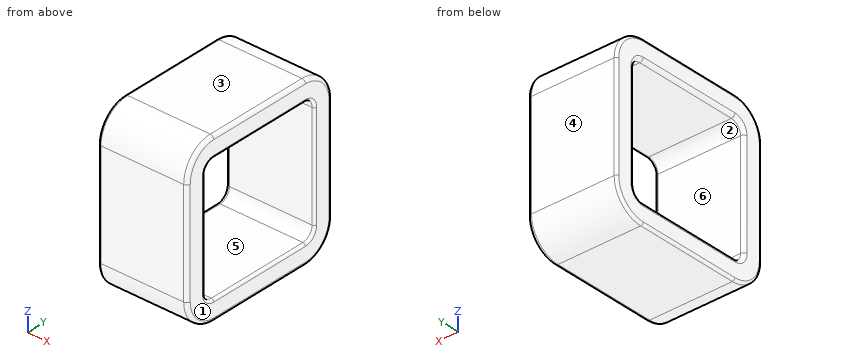
```python
from build123d import *

# Parameters (mm, degrees)
BOSS_EXTRUDE1_DEPTH      = 12
BOSS_EXTRUDE1_DEPTH_BACK = 5.8
FILLET2_R                = 0.7
FILLET3_R                = 0.5


with BuildPart() as part:
    # Sketch1 → Boss-Extrude1 (new, two sides: drawn at the far end of the back side and taken through both)
    with BuildSketch(Plane(origin=(72.6, 0, 0), x_dir=(0, 0, -1), z_dir=(1, 0, 0)).offset(-BOSS_EXTRUDE1_DEPTH_BACK)):
        with BuildLine():
            Line((-31.6, 17.5), (-31.6, -3.5))
            ThreePointArc((-31.6, -3.5), (-29.813351365, -7.813351365), (-25.5, -9.6))
            Line((-25.5, -9.6), (-4.5, -9.6))
            ThreePointArc((-4.5, -9.6), (-0.186648635, -7.813351365), (1.6, -3.5))
            Line((1.6, -3.5), (1.6, 17.5))
            ThreePointArc((1.6, 17.5), (-0.186648635, 21.813351365), (-4.5, 23.6))
            Line((-4.5, 23.6), (-25.5, 23.6))
            ThreePointArc((-25.5, 23.6), (-29.813351365, 21.813351365), (-31.6, 17.5))
        make_face()
        with BuildLine():
            Line((-27.6, 17.5), (-27.6, -3.5))
            ThreePointArc((-27.6, -3.5), (-26.98492424, -4.98492424), (-25.5, -5.6))
            Line((-25.5, -5.6), (-4.5, -5.6))
            ThreePointArc((-4.5, -5.6), (-3.01507576, -4.98492424), (-2.4, -3.5))
            Line((-2.4, -3.5), (-2.4, 17.5))
            ThreePointArc((-2.4, 17.5), (-3.01507576, 18.98492424), (-4.5, 19.6))
            Line((-4.5, 19.6), (-25.5, 19.6))
            ThreePointArc((-25.5, 19.6), (-26.98492424, 18.98492424), (-27.6, 17.5))
        make_face(mode=Mode.SUBTRACT)
    extrude(amount=BOSS_EXTRUDE1_DEPTH + BOSS_EXTRUDE1_DEPTH_BACK)

    # Fillet2
    fillet2_edges = [part.edges().sort_by_distance(p)[0] for p in [
        (66.8, 18.98492424, 26.98492424),
        (66.8, 7, 27.6),
        (66.8, -4.98492424, 26.98492424),
        (66.8, -5.6, 15),
        (84.6, 23.6, 15),
        (66.8, -4.98492424, 3.01507576),
        (66.8, 18.98492424, 3.01507576),
        (84.6, 21.813351365, 29.813351365),
        (66.8, 7, 2.4),
        (66.8, 19.6, 15),
        (84.6, 7, 31.6),
        (84.6, -7.813351365, 29.813351365),
        (84.6, -9.6, 15),
        (84.6, -7.813351365, 0.186648635),
        (84.6, 7, -1.6),
        (84.6, 21.813351365, 0.186648635),
    ]]
    fillet(fillet2_edges, radius=FILLET2_R)

    # Fillet3
    fillet3_edges = [part.edges().sort_by_distance(p)[0] for p in [
        (84.6, 19.6, 15),
        (84.6, 18.98492424, 3.01507576),
        (84.6, 7, 2.4),
        (84.6, -4.98492424, 3.01507576),
        (84.6, -5.6, 15),
        (84.6, -4.98492424, 26.98492424),
        (84.6, 7, 27.6),
        (66.8, 23.6, 15),
        (66.8, 7, -1.6),
        (66.8, 21.813351365, 0.186648635),
        (66.8, -7.813351365, 0.186648635),
        (66.8, -9.6, 15),
        (66.8, -7.813351365, 29.813351365),
        (66.8, 7, 31.6),
        (66.8, 21.813351365, 29.813351365),
        (84.6, 18.98492424, 26.98492424),
    ]]
    fillet(fillet3_edges, radius=FILLET3_R)


solid = part.part
```
The listing builds one solid part. Answer for the finished solid, in the listing's coordinates (mm). Face numbers are marked on the shaded views. A direction names the side the tool comes from. Give positions to 0.01 mm unless a question says otherwise; leave off trailing zeros. Write each loop counter-clockwise with the first axis right and the second up, starting at its lowest first coordinate (ties: lowest second). Pieces come first, ordered by that corner, then holes. Notation, with made-up numbers: M -24.75,18.25 L -9.75,18.25 A32 cw -9.75,52.25 Z; hole C -35.75,67.25 d10. An arc over 180 degrees is marked long. Write each question's results on one line, items separated by ' | '.
Q1. A tool of negligible diameter and unlimited length cuts with its end or side. For the marked faces 1 and 2, from which of +Z, -Z, +X, -X, +Y, -Y can it reach the whole face along a straight path? Write none if from no direction.
Output values:
face 1: +Z, -Z, +X, +Y, -Y | face 2: +X, -X
Q2. Flat-ended cylindrical pins translate along their axes: P1, Ø1, axis at x = 77, y = -5.5, coming from the +Z side; P2, Ø5, axis at y = 17.5, z = 8.5, coming from the +X side. Find the tip coordinate at first contact, or state that the pin passes through.
Output values:
P1: z = 31.41 | P2: x = 84.59
Q3. Section C-C, the plane z = 14.5 is taken. Write down the section's boundary in (x, y).
Output values:
outline: M 66.8,-9.1 A0.5 ccw 67.3,-9.6 L 83.9,-9.6 A0.7 ccw 84.6,-8.9 L 84.6,-6.1 A0.5 ccw 84.1,-5.6 L 67.5,-5.6 A0.7 ccw 66.8,-6.3 Z; M 66.8,20.3 A0.7 ccw 67.5,19.6 L 84.1,19.6 A0.5 ccw 84.6,20.1 L 84.6,22.9 A0.7 ccw 83.9,23.6 L 67.3,23.6 A0.5 ccw 66.8,23.1 Z
Q4. Section B-B, the plane x = 68.75 is taken. Write down the section's boundary in (y, z).
Output values:
outline: M -9.6,4.5 A6.1 ccw -3.5,-1.6 L 17.5,-1.6 A6.1 ccw 23.6,4.5 L 23.6,25.5 A6.1 ccw 17.5,31.6 L -3.5,31.6 A6.1 ccw -9.6,25.5 Z; hole M -5.6,4.5 A2.1 ccw -3.5,2.4 L 17.5,2.4 A2.1 ccw 19.6,4.5 L 19.6,25.5 A2.1 ccw 17.5,27.6 L -3.5,27.6 A2.1 ccw -5.6,25.5 Z
Q5. Consider L1, parallel to Y at x = 74.75, z = 15.5; L2, parallel to Z at x = 69, y = -1; L3, parallel to Z at x = 84.25, y = 13.5. Determine where each line is inside the solid, lowest interval first. Write a range as from..to.
Output values:
L1: -9.6..-5.6, 19.6..23.6 | L2: -1.6..2.4, 27.6..31.6 | L3: -1.51..2.38, 27.62..31.51
Q6. For a pull along Y with two mould halves and no side action, classify the marked faces 3, 4, 5 and 6 as released by +Y, released by -Y, zero draft, split by the parting line, or undercut.
Output values:
face 3: zero draft | face 4: released by +Y | face 5: undercut | face 6: undercut
Q7. Section A-A, the plane y = 4 is taken. Write down the section's boundary in (x, z), then the cut area to 3 significant figures.
Output values:
outline: M 66.8,-1.1 A0.5 ccw 67.3,-1.6 L 83.9,-1.6 A0.7 ccw 84.6,-0.9 L 84.6,1.9 A0.5 ccw 84.1,2.4 L 67.5,2.4 A0.7 ccw 66.8,1.7 Z; M 66.8,28.3 A0.7 ccw 67.5,27.6 L 84.1,27.6 A0.5 ccw 84.6,28.1 L 84.6,30.9 A0.7 ccw 83.9,31.6 L 67.3,31.6 A0.5 ccw 66.8,31.1 Z | area: 142 mm2
